Source: CAD feature listing. Evaluate the final solid. Frame: model axes, mm. A direction names the side the tool comes from. Give positions to 0.01 mm unless a question says otherwise; leave off trailing zeros. Order: outer loops, then holes, each group sorted by start corner. A loop starts at its lowest first (then second) coordinate and runs counter-clockwise, first axis right, second up.
```python
from build123d import *

# Parameters (mm, degrees)
BOSS_EXTRUDE1_DEPTH          = 127
F_12_5_12_5_DIAMETER_HOLE1_D = 12.5
F_12_5_12_5_DIAMETER_HOLE2_D = 12.5


with BuildPart() as part:
    # Sketch1 → Boss-Extrude1 (new body)
    with BuildSketch(Plane.XY):
        Polygon((54.15, -35.1), (54.15, 38.1), (57.15, 38.1), (57.15, -38.1), (-57.15, -38.1), (-57.15, 38.1), (-54.15, 38.1), (-54.15, -35.1), align=None)
    extrude(amount=BOSS_EXTRUDE1_DEPTH)

    # Ø12.5 (12.5) Diameter Hole1 (through all)
    with Locations(Plane(origin=(0, -35.1, 0), x_dir=(1, 0, 0), z_dir=(0, 1, 0))):
        with Locations((0, -63.5)):
            Hole(F_12_5_12_5_DIAMETER_HOLE1_D / 2)

    # Ø12.5 (12.5) Diameter Hole2 (through all)
    with Locations(Plane.ZY.offset(57.15)):
        with Locations((63.5, 0)):
            Hole(F_12_5_12_5_DIAMETER_HOLE2_D / 2)


solid = part.part
```
1) Pin query (flat end, axial travel): pin 1 (12 mm diameter, centred on x = 26.5, z = 77.5, fed in from +Y). Return the tip coordinate at first contact, or that it passes through.
Report:
pin 1: stops at y = -35.1
2) Material intervals for L1, parallel to Y at x = -54.8, z = 63.5; L2, parallel to X at y = 12.5, z = 39.5; L3, parallel to X at y = -36, z = 63, sorted ascending.
Report:
L1: y = -38.1 to -6.25, 6.25 to 38.1
L2: x = -57.15 to -54.15, 54.15 to 57.15
L3: x = -57.15 to -6.23, 6.23 to 57.15
3) Section query C-C, the plane z = 63.5. Return the cut outline in (x, y).
Report:
outline: (-57.15, -38.1) - (-6.25, -38.1) - (-6.25, -35.1) - (-54.15, -35.1) - (-54.15, -6.25) - (-57.15, -6.25) - close; (-57.15, 6.25) - (-54.15, 6.25) - (-54.15, 38.1) - (-57.15, 38.1) - close; (6.25, -38.1) - (57.15, -38.1) - (57.15, -6.25) - (54.15, -6.25) - (54.15, -35.1) - (6.25, -35.1) - close; (54.15, 6.25) - (57.15, 6.25) - (57.15, 38.1) - (54.15, 38.1) - close
4) Section query D-D, the plane y = 0. Return the cut outline in (x, z), and give its area (3 significant figures).
Report:
outline: (-57.15, 0) - (-54.15, 0) - (-54.15, 57.25) - (-57.15, 57.25) - close; (-57.15, 69.75) - (-54.15, 69.75) - (-54.15, 127) - (-57.15, 127) - close; (54.15, 0) - (57.15, 0) - (57.15, 57.25) - (54.15, 57.25) - close; (54.15, 69.75) - (57.15, 69.75) - (57.15, 127) - (54.15, 127) - close
area: 687 mm2
5) Draft query along Z for faces 1 (the flat face through (-12, -38.1, 63)), 2 (the cylindrical face through (55.67, 1.88, 57.54)), 3 (the flat face through (0, -37, 127)). Return one class per face: +Z half, -Z half, draft (parallel to the pull), parting line (faces both ways), or undercut.
Report:
face 1: draft
face 2: undercut
face 3: +Z half
6) Section query A-A, the plane y = -15. Return the cut outline in (x, z).
Report:
outline: (-57.15, 0) - (-54.15, 0) - (-54.15, 127) - (-57.15, 127) - close; (54.15, 0) - (57.15, 0) - (57.15, 127) - (54.15, 127) - close
7) Reachability of faces 4 (the flat face through (-56, 38.1, 63)), 5 (the flat face through (-54.15, 10, 63)) from +Z, -Z, +X, -X, +Y, -Y: full face, straight path, thin tool, end or side. Return the list, or none.
Report:
face 4: +Z, -Z, +X, -X, +Y
face 5: +Z, -Z, +Y
8) Section query B-B, the plane x = 0. Return the cut outline in (y, z).
Report:
outline: (-38.1, 0) - (-35.1, 0) - (-35.1, 57.25) - (-38.1, 57.25) - close; (-38.1, 69.75) - (-35.1, 69.75) - (-35.1, 127) - (-38.1, 127) - close
